Here's how the part is built. I have some questions about the finished solid (model axes, mm). Coordinates: 2 decimals unless noted, no trailing zeros. Write each loop counter-clockwise with the first axis right and the second up, starting at its lowest first coordinate (ties: lowest second). Pieces come first, ordered by that corner, then holes. Notation, with made-up numbers: (-26, -29) -> (8, -29) arc R29 cw to (8, 9) -> close; hole circle Ø10 at (-7, 58). An arc over 180 degrees is marked (long way). Answer in a Markdown table with one row per item. Add a question column.
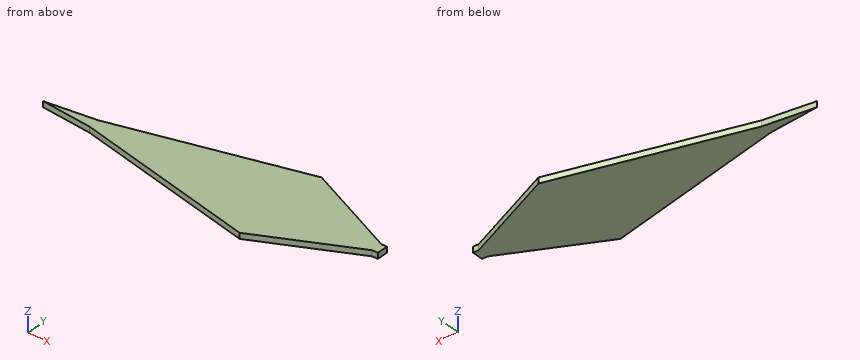
from build123d import *

# Parameters (mm, degrees)
F0_W     = 9.6744340956
F0_H     = 1
F1_DEPTH = 1


# Not quite as in the source:
# - a feature names something its author has since deleted; it is built from what else it names


with BuildPart() as f1:
    # F0 (on Top) → F1 (new body)
    with BuildSketch(Plane.XY):
        with Locations((-20.6627829522, 0.5)):
            Rectangle(F0_W, F0_H)
        Polygon((-34.5, 0), (-25.5, 0), (-25.5, 1), align=None)
        Polygon((-15.8255659044, 0), (-25.5, 0), (-25.5, -1), (24.5, -1), (25.5, -1), (25.5, 0), align=None)
        Polygon((-25.5, -1), (-25.5, 0), (-34.5, 0), align=None)
        Polygon((-15.8255659044, 1), (-15.8255659044, 0), (25.5, 0), (25.5, 1), (24.5, 1), align=None)
        with BuildLine():
            add(Edge.make_bspline(
                [(-25.5, 1), (-14.5003329962, 3.3801647369), (-13.2050132379, 2.5), (7.5, 3)],
                knots=[0, 0, 0, 0, 33.0605505096, 33.0605505096, 33.0605505096, 33.0605505096], degree=3))
            Line((-25.5, 1), (-15.8255659044, 1))
            Line((-15.8255659044, 1), (24.5, 1))
            add(Edge.make_bspline(
                [(7.5, 3), (14.1289979219, 2.5626332499), (18.8218969852, 1.9759975839), (24.5, 1)],
                knots=[0, 0, 0, 0, 17.1172427686, 17.1172427686, 17.1172427686, 17.1172427686], degree=3))
        make_face()
        with BuildLine():
            Line((7.5, 9), (-25.5, 1))
            add(Edge.make_bspline(
                [(-25.5, 1), (-14.5003329962, 3.3801647369), (-13.2050132379, 2.5), (7.5, 3)],
                knots=[0, 0, 0, 0, 33.0605505096, 33.0605505096, 33.0605505096, 33.0605505096], degree=3))
            add(Edge.make_bspline(
                [(7.5, 3), (14.1289979219, 2.5626332499), (18.8218969852, 1.9759975839), (24.5, 1)],
                knots=[0, 0, 0, 0, 17.1172427686, 17.1172427686, 17.1172427686, 17.1172427686], degree=3))
            Line((24.5, 1), (7.5, 9))
        make_face()
        with BuildLine():
            add(Edge.make_bspline(
                [(-25.5, -1), (-14.5003329962, -3.3801647369), (-13.2050132379, -2.5), (7.5, -3)],
                knots=[0, 0, 0, 0, 33.0605505096, 33.0605505096, 33.0605505096, 33.0605505096], degree=3))
            Line((-25.5, -1), (7.5, -9))
            Line((7.5, -9), (24.5, -1))
            add(Edge.make_bspline(
                [(7.5, -3), (14.1289979219, -2.5626332499), (18.8218969852, -1.9759975839), (24.5, -1)],
                knots=[0, 0, 0, 0, 17.1172427686, 17.1172427686, 17.1172427686, 17.1172427686], degree=3))
        make_face()
        with BuildLine():
            Line((24.5, -1), (-25.5, -1))
            add(Edge.make_bspline(
                [(-25.5, -1), (-14.5003329962, -3.3801647369), (-13.2050132379, -2.5), (7.5, -3)],
                knots=[0, 0, 0, 0, 33.0605505096, 33.0605505096, 33.0605505096, 33.0605505096], degree=3))
            add(Edge.make_bspline(
                [(7.5, -3), (14.1289979219, -2.5626332499), (18.8218969852, -1.9759975839), (24.5, -1)],
                knots=[0, 0, 0, 0, 17.1172427686, 17.1172427686, 17.1172427686, 17.1172427686], degree=3))
        make_face()
    extrude(amount=F1_DEPTH)


solid = f1.part
Q1. I'm going to push flat-ended pins straight in: P1, Ø1, axis at x = -22, y = 0, coming from the -Z side; P2, Ø0.5, axis at x = 25, z = 0.5, coming from the +Y side. Where does each tip first touch, or does it pass through?
Q2. Imagine slicing it at C-C on x = -16.5. Please give me the cut outline in (y, z).
Q3. Imagine slicing it at A-A on z = 0.65. Please give me the cut outline in (x, y), plus the area to 3 significant figures.
Q4. Imagine slicing it at B-B on y = -3. Please give me the cut outline in (x, z), plus the area to 3 significant figures.
Q5. I need wall thicknesses on line 1 (Y direction, x = -27.5, z = 0.95); line 2 (Y direction, x = -22, z = 0.2). Which ranges of each line are inside material? Lowest first, please. Write a range as [from, to].
Result sheet:
| question | item | result |
|---|---|---|
| 1 | P1 | stops at z = 0 |
| 1 | P2 | stops at y = 1 |
| 2 | outline | (-3.18, 0) -> (3.18, 0) -> (3.18, 1) -> (-3.18, 1) -> close |
| 3 | outline | (-34.5, 0) -> (-25.5, -1) -> (7.5, -9) -> (24.5, -1) -> (25.5, -1) -> (25.5, 1) -> (24.5, 1) -> (7.5, 9) -> (-25.5, 1) -> close |
| 3 | area | 511 mm^2 |
| 4 | outline | (-17.25, 0) -> (20.25, 0) -> (20.25, 1) -> (-17.25, 1) -> close |
| 4 | area | 37.5 mm^2 |
| 5 | line 1 | y = [-0.78, 0.78] |
| 5 | line 2 | y = [-1.85, 1.85] |
